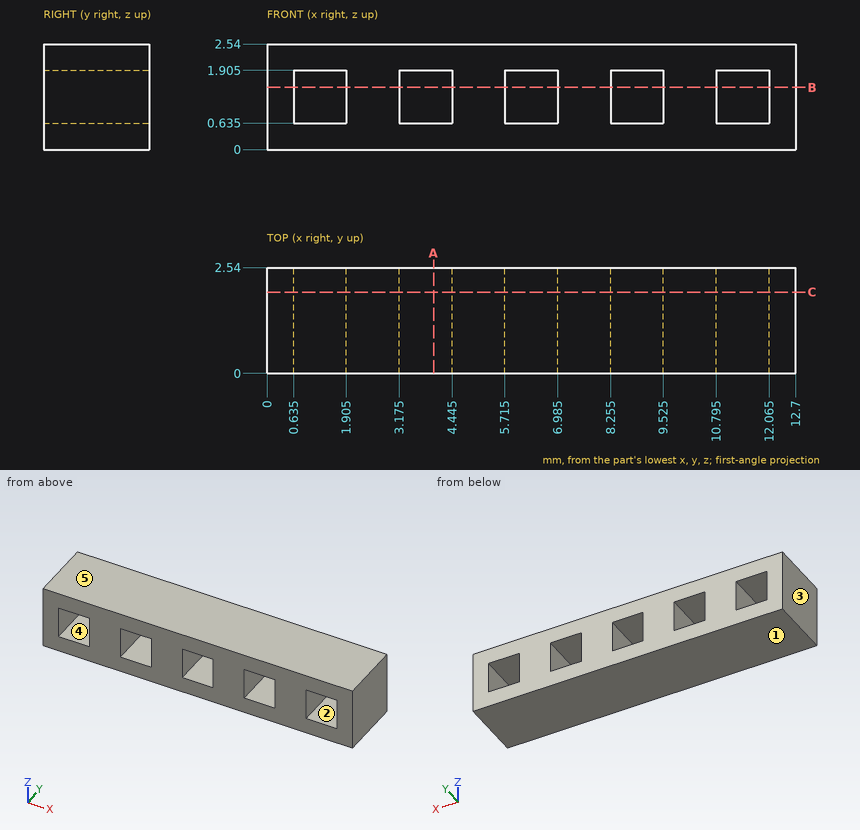
The drawing under review shows one solid part. Ordinate dimensions are in mm from its lowest x, y, z. A direction names the side the tool comes from. Give positions to 0.01 mm unless a question says otherwise; leave off trailing zeros. Write each loop counter-clockwise with the first axis right and the second up, starting at its lowest first coordinate (ties: lowest second). Pieces come first, ordered by that corner, then holes.
1. Draft analysis for pull direction X (two halves, no side actions). For the marked faces 3, 4 and 5, state which applies: +X half, -X half, draft (parallel to the pull), parting line (faces both ways), or undercut.
2. For P1, Ø1.4, axis at y = 1, z = 1, coming from the -X side, flat-tipped, find the tip position at first contact; note if it passes through.
3. Add section A-A, the plane x = 4. Write out the cut boundary in (y, z) (3 decimals).
4. Tool access review of the marked faces 1 and 2: name each direction out of +Z, -Z, +X, -X, +Y, -Y from which nothing blocks a thin tool from reaching the whole face with its end or side.
5. Wall thickness on L1, parallel to X at y = 1.25, z = 1.2 (3 decimals); L2, parallel to Z at x = 6.75, y = 1.35 (3 decimals): over which ranges is each line inside the solid? List them lowest first.
6. Add section C-C, the plane y = 1.95. Write out the cut boundary in (x, z) (3 decimals).
7. Add section B-B, the plane z = 1.5. Write out the cut boundary in (x, y) (3 decimals), plus the area to 3 significant figures.
Worked answers:
1. face 3: -X half
1. face 4: undercut
1. face 5: draft
2. P1: stops at x = 0
3. outline: (0, 0) - (2.54, 0) - (2.54, 0.635) - (0, 0.635) - close; (0, 1.905) - (2.54, 1.905) - (2.54, 2.54) - (0, 2.54) - close
4. face 1: -Z, +X, -X, +Y, -Y
4. face 2: +Y, -Y
5. L1: x = 0 to 0.635, 1.905 to 3.175, 4.445 to 5.715, 6.985 to 8.255, 9.525 to 10.795, 12.065 to 12.7
5. L2: z = 0 to 0.635, 1.905 to 2.54
6. outline: (0, 0) - (12.7, 0) - (12.7, 2.54) - (0, 2.54) - close; hole (0.635, 0.635) - (1.905, 0.635) - (1.905, 1.905) - (0.635, 1.905) - close; hole (3.175, 0.635) - (4.445, 0.635) - (4.445, 1.905) - (3.175, 1.905) - close; hole (5.715, 0.635) - (6.985, 0.635) - (6.985, 1.905) - (5.715, 1.905) - close; hole (8.255, 0.635) - (9.525, 0.635) - (9.525, 1.905) - (8.255, 1.905) - close; hole (10.795, 0.635) - (12.065, 0.635) - (12.065, 1.905) - (10.795, 1.905) - close
7. outline: (0, 0) - (0.635, 0) - (0.635, 2.54) - (0, 2.54) - close; (1.905, 0) - (3.175, 0) - (3.175, 2.54) - (1.905, 2.54) - close; (4.445, 0) - (5.715, 0) - (5.715, 2.54) - (4.445, 2.54) - close; (6.985, 0) - (8.255, 0) - (8.255, 2.54) - (6.985, 2.54) - close; (9.525, 0) - (10.795, 0) - (10.795, 2.54) - (9.525, 2.54) - close; (12.065, 0) - (12.7, 0) - (12.7, 2.54) - (12.065, 2.54) - close
7. area: 16.1 mm2
